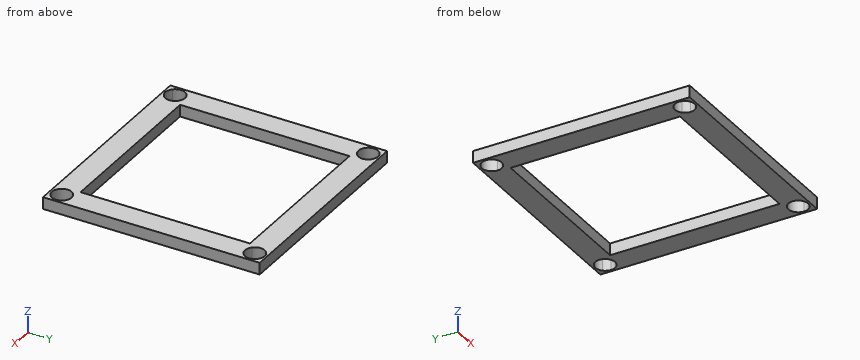
```python
from build123d import *

# Parameters (mm, degrees)
F1_DEPTH = 3


with BuildPart() as f1:
    # F0 (on Top) → F1 (new body)
    with BuildSketch(Plane.XY):
        with BuildLine():
            Line((-26.267767, 26.267767), (-27.5, 27.5))
            Line((-27.5, 27.5), (-27.5, -27.5))
            Line((-27.5, -27.5), (-26.267767, -26.267767))
            ThreePointArc((-26.267767, -26.267767), (-26.267767, -22.732233), (-22.732233, -22.732233))
            Line((-22.732233, -22.732233), (-21.5, -21.5))
            Line((-21.5, -21.5), (-21.5, 21.5))
            Line((-21.5, 21.5), (-22.732233, 22.732233))
            ThreePointArc((-22.732233, 22.732233), (-26.267767, 22.732233), (-26.267767, 26.267767))
        make_face()
        with BuildLine():
            Line((-27.5, -27.5), (27.5, -27.5))
            Line((27.5, -27.5), (26.267767, -26.267767))
            ThreePointArc((26.267767, -26.267767), (22.732233, -26.267767), (22.732233, -22.732233))
            Line((22.732233, -22.732233), (21.5, -21.5))
            Line((21.5, -21.5), (-21.5, -21.5))
            Line((-21.5, -21.5), (-22.732233, -22.732233))
            ThreePointArc((-22.732233, -22.732233), (-22.190301, -23.543291), (-22, -24.5))
            ThreePointArc((-22, -24.5), (-23.543291, -26.809699), (-26.267767, -26.267767))
            Line((-26.267767, -26.267767), (-27.5, -27.5))
        make_face()
        with BuildLine():
            Line((27.5, -27.5), (27.5, 27.5))
            Line((27.5, 27.5), (26.267767, 26.267767))
            ThreePointArc((26.267767, 26.267767), (26.809699, 25.456709), (27, 24.5))
            ThreePointArc((27, 24.5), (25.456709, 22.190301), (22.732233, 22.732233))
            Line((22.732233, 22.732233), (21.5, 21.5))
            Line((21.5, 21.5), (21.5, -21.5))
            Line((21.5, -21.5), (22.732233, -22.732233))
            ThreePointArc((22.732233, -22.732233), (25.456709, -22.190301), (27, -24.5))
            ThreePointArc((27, -24.5), (26.809699, -25.456709), (26.267767, -26.267767))
            Line((26.267767, -26.267767), (27.5, -27.5))
        make_face()
        with BuildLine():
            Line((26.267767, 26.267767), (27.5, 27.5))
            Line((27.5, 27.5), (-27.5, 27.5))
            Line((-27.5, 27.5), (-26.267767, 26.267767))
            ThreePointArc((-26.267767, 26.267767), (-23.543291, 26.809699), (-22, 24.5))
            ThreePointArc((-22, 24.5), (-22.190301, 23.543291), (-22.732233, 22.732233))
            Line((-22.732233, 22.732233), (-21.5, 21.5))
            Line((-21.5, 21.5), (21.5, 21.5))
            Line((21.5, 21.5), (22.732233, 22.732233))
            ThreePointArc((22.732233, 22.732233), (22.732233, 26.267767), (26.267767, 26.267767))
        make_face()
    extrude(amount=F1_DEPTH)


solid = f1.part
```
Design review of the part built by this model. Coordinates are the model's own, in mm. Coordinates: 2 decimals unless noted, no trailing zeros. Write each loop counter-clockwise with the first axis right and the second up, starting at its lowest first coordinate (ties: lowest second). Pieces come first, ordered by that corner, then holes.
1) Add section A-A (x = -24.5). Write out the cut boundary in (y, z), plus the area to 3 significant figures.
2) To check wall thickness, follow L1, parallel to Y at x = -8.5, z = 0.8; L2, parallel to X at y = 24, z = 1.75. State the ranges of each line that lie inside material, in increasing order.
3) Add section D-D (z = 2.25). Write out the cut boundary in (x, y), plus the area to 3 significant figures.
4) Add section B-B (y = 12). Write out the cut boundary in (x, z).
Check result:
1. outline: (-27.5, 0) - (-27, 0) - (-27, 3) - (-27.5, 3) - close; (-22, 0) - (22, 0) - (22, 3) - (-22, 3) - close; (27, 0) - (27.5, 0) - (27.5, 3) - (27, 3) - close
1. area: 135 mm2
2. L1: y = -27.5 to -21.5, 21.5 to 27.5
2. L2: x = -27.5 to -26.95, -22.05 to 22.05, 26.95 to 27.5
3. outline: (-27.5, -27.5) - (27.5, -27.5) - (27.5, 27.5) - (-27.5, 27.5) - close; hole (-22.73, -22.73) arc R2.5 ccw (long way) to (-22, -24.5) arc R2.5 ccw to start; hole (-22.73, 22.73) arc R2.5 ccw to (-22, 24.5) arc R2.5 ccw (long way) to start; hole (-21.5, -21.5) - (21.5, -21.5) - (21.5, 21.5) - (-21.5, 21.5) - close; hole (26.27, -26.27) arc R2.5 ccw to (27, -24.5) arc R2.5 ccw (long way) to start; hole (26.27, 26.27) arc R2.5 ccw (long way) to (27, 24.5) arc R2.5 ccw to start
3. area: 1,100 mm2
4. outline: (-27.5, 0) - (-21.5, 0) - (-21.5, 3) - (-27.5, 3) - close; (21.5, 0) - (27.5, 0) - (27.5, 3) - (21.5, 3) - close
